from build123d import *

# Parameters (mm, degrees)
F0_W     = 49.706
F0_H     = 50
F1_DEPTH = 1
F2_R     = 2.25
F3_DEPTH = 5
F4_R     = 5
F5_DEPTH = 25


with BuildPart() as f1:
    # F0 (on Top) → F1 (new body)
    with BuildSketch(Plane.XY):
        Rectangle(F0_W, F0_H)
    extrude(amount=F1_DEPTH)

    # F2 (on face) → F3 (join)
    with BuildSketch(Plane.XY.offset(1)):
        with Locations((-12, 12)):
            Circle(F2_R)
        with Locations((12, 12)):
            Circle(F2_R)
        with Locations((-12, -12)):
            Circle(F2_R)
        with Locations((12, -12)):
            Circle(F2_R)
    extrude(amount=F3_DEPTH)

    # F4 (on face) → F5 (cut)
    with BuildSketch(Plane.XY.offset(1)):
        Circle(F4_R)
    extrude(amount=-F5_DEPTH, mode=Mode.SUBTRACT)


solid = f1.part
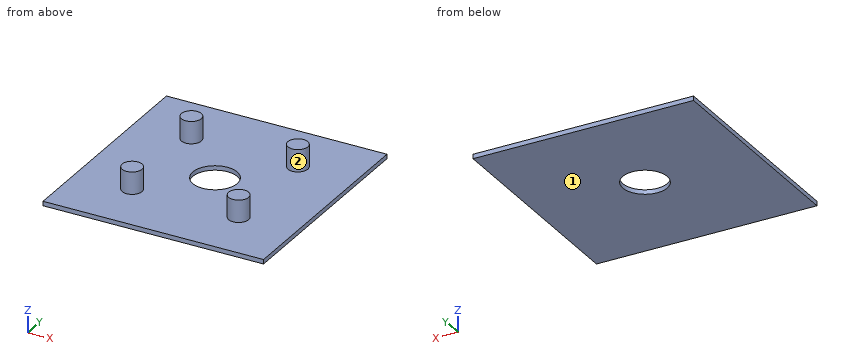
Geometry: final body of the model. Coordinates: model frame, mm. Face numbers are marked on the shaded views. Round coordinates to 2 decimals unless told otherwise and drop trailing zeros. Order: outer loops, then holes, each group sorted by start corner. A loop starts at its lowest first (then second) coordinate and runs counter-clockwise, first axis right, second up.
Q1. Material intervals for probe 1 along Y at (x, z) = (0, 0.75); probe 2 along Z at (x, y) = (-8, 22.5); probe 3 along X at (y, z) = (-13, 2.6), sorted ascending.
Result sheet:
probe 1: y = -25 to -5, 5 to 25
probe 2: z = 0 to 1
probe 3: x = -14.02 to -9.98, 9.98 to 14.02
Q2. Section B-B, the plane y = 0. Output: boundary loops of the cut face in (x, z).
Result sheet:
outline: (-24.85, 0) - (-5, 0) - (-5, 1) - (-24.85, 1) - close; (5, 0) - (24.85, 0) - (24.85, 1) - (5, 1) - close
Q3. Section D-D, the plane z = 1.95. Output: boundary loops of the cut face in (x, y).
Result sheet:
outline: circle Ø4.5 at (-12, -12); circle Ø4.5 at (-12, 12); circle Ø4.5 at (12, -12); circle Ø4.5 at (12, 12)
Q4. Section C-C, the plane x = -12. Output: boundary loops of the cut face in (y, z), and give its area (3 significant figures).
Result sheet:
outline: (-25, 0) - (25, 0) - (25, 1) - (14.25, 1) - (14.25, 6) - (9.75, 6) - (9.75, 1) - (-9.75, 1) - (-9.75, 6) - (-14.25, 6) - (-14.25, 1) - (-25, 1) - close
area: 95.0 mm2
Q5. Section A-A, the plane x = 3. Output: boundary loops of the cut face in (y, z), and give its area (3 significant figures).
Result sheet:
outline: (-25, 0) - (-4, 0) - (-4, 1) - (-25, 1) - close; (4, 0) - (25, 0) - (25, 1) - (4, 1) - close
area: 42.0 mm2
Q6. Mould query, pull axis Y, two halves, no side actions, for the marked faces 1 and 2. Classes: released by +Y, released by -Y, zero draft, split by the parting line, or undercut.
Result sheet:
face 1: zero draft
face 2: undercut
Q7. Pin query (flat end, axial travel): pin 1 (25 mm diameter, centred on x = -8.5, y = -5, fed in from +Z); pin 2 (4 mm diameter, centred on x = -9, y = 1, fed in from +Z); pin 3 (1.5 mm diameter, centred on y = 6, z = 3, fed in from +X). Return the tip coordinate at first contact, or that it passes through.
Result sheet:
pin 1: stops at z = 6
pin 2: stops at z = 1
pin 3: passes through
